Can you work these out from the model? Positions are in its coordinate system, mm. Coordinates: 2 decimals unless noted, no trailing zeros. Order: outer loops, then holes, each group sorted by start corner. A loop starts at its lowest first (then second) coordinate and runs counter-clockwise, first axis right, second up. Notation, with made-up numbers: (60.5, 1.25) -> (102.5, 1.25) arc R20 ccw to (102.5, 26.25) -> close; hole circle Ø9 at (64, 29.5). An arc over 180 degrees is marked (long way). Answer in a Markdown table with one row per item. Add a question column.
1. If I drill on line 1 along Y through (x, z) = (41.7, 1.6); line 2 along X through (y, z) = (5.5, 0.65); line 3 along Y through (x, z) = (42.5, 0.95), over which ranges is the centre line in solid material (lowest first)? Write a range as [from, to].
2. Imagine slicing it at C-C on x = 24. Write out the boundary of the cut face in (y, z), plus the area to 3 significant figures.
3. Imagine slicing it at D-D on z = 1.4. Write out the boundary of the cut face in (x, y), plus the area to 3 significant figures.
4. Imagine slicing it at B-B on x = 31.5. Write out the boundary of the cut face in (y, z).
5. Will these pins go through, and if not, where does the flat tip stop? pin 1 (1.5 mm diameter, centred on x = 5, y = 24.5, fed in from +Z); pin 2 (0.9 mm diameter, centred on x = 36.5, z = 2, fed in from -Y); pin 3 (1.5 mm diameter, centred on y = 30, z = 1, fed in from -X); pin 4 (1.5 mm diameter, centred on y = 21.5, z = 1.5, fed in from -X).
6. Imagine slicing it at A-A on x = 41.7. Write out the boundary of the cut face in (y, z).
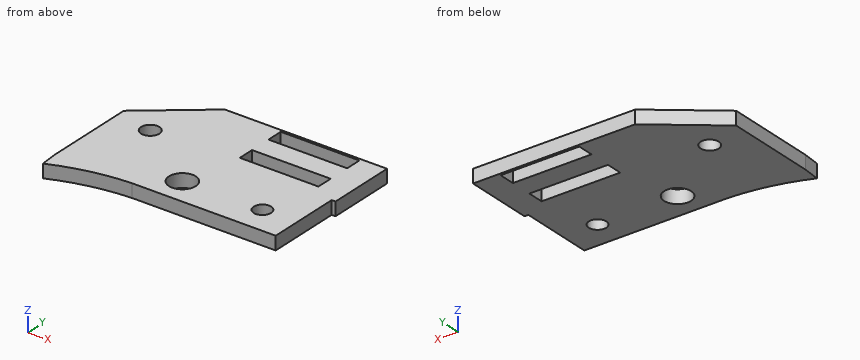
from build123d import *

# Parameters (mm, degrees)
SKETCH_1_R      = 3
SKETCH_1_R_2    = 1.95
SKETCH_1_R_3    = 2.05
SKETCH_1_W      = 17.535566723
SKETCH_1_H      = 3.6
EXTRUDE_1_DEPTH = 3


with BuildPart() as part:
    # 스케치1 → 보스-돌출1 (new body)
    with BuildSketch(Plane.XY):
        with BuildLine():
            Line((14.033980913, 31.631973376), (0, 20.408728084))
            Line((0, 20.408728084), (0, 0))
            Line((0, 0), (0.315433782, -3.780966668))
            ThreePointArc((0.315433782, -3.780966668), (8.660717355, -1.110252043), (17.352311853, 0))
            Line((17.352311853, 0), (49.356011681, 0))
            Line((49.356011681, 0), (49.356011681, 16.484705835))
            Line((49.356011681, 16.484705835), (50.213133896, 16.484705835))
            Line((50.213133896, 16.484705835), (50.213133896, 31.631973376))
            Line((50.213133896, 31.631973376), (14.033980913, 31.631973376))
        make_face()
        with Locations((24, 6)):
            Circle(SKETCH_1_R, mode=Mode.SUBTRACT)
        with Locations((41.7, 6.2)):
            Circle(SKETCH_1_R_2, mode=Mode.SUBTRACT)
        with Locations((8.103885944, 17.512168243)):
            Circle(SKETCH_1_R_3, mode=Mode.SUBTRACT)
        with Locations((35.691910847, 29.288073102)):
            Rectangle(SKETCH_1_W, SKETCH_1_H, mode=Mode.SUBTRACT)
        with Locations((35.691910847, 20.838073102)):
            Rectangle(SKETCH_1_W, SKETCH_1_H, mode=Mode.SUBTRACT)
    extrude(amount=EXTRUDE_1_DEPTH)


solid = part.part
Answers follow:
| question | item | result |
|---|---|---|
| 1 | line 1 | y = [0, 4.25], [8.15, 19.04], [22.64, 27.49], [31.09, 31.63] |
| 1 | line 2 | x = [0, 21.04], [26.96, 39.88], [43.52, 49.36] |
| 1 | line 3 | y = [0, 4.42], [7.98, 19.04], [22.64, 27.49], [31.09, 31.63] |
| 2 | outline | (0, 0) -> (3, 0) -> (3, 3) -> (0, 3) -> close; (9, 0) -> (31.63, 0) -> (31.63, 3) -> (9, 3) -> close |
| 2 | area | 76.9 mm² |
| 3 | outline | (0, 0) -> (0.32, -3.78) arc R48.03 cw to (17.35, 0) -> (49.36, 0) -> (49.36, 16.48) -> (50.21, 16.48) -> (50.21, 31.63) -> (14.03, 31.63) -> (0, 20.41) -> close; hole circle Ø4.1 at (8.1, 17.51); hole circle Ø6 at (24, 6); hole (26.92, 19.04) -> (44.46, 19.04) -> (44.46, 22.64) -> (26.92, 22.64) -> close; hole (26.92, 27.49) -> (44.46, 27.49) -> (44.46, 31.09) -> (26.92, 31.09) -> close; hole circle Ø3.9 at (41.7, 6.2) |
| 3 | area | 1,340 mm² |
| 4 | outline | (0, 0) -> (19.04, 0) -> (19.04, 3) -> (0, 3) -> close; (22.64, 0) -> (27.49, 0) -> (27.49, 3) -> (22.64, 3) -> close; (31.09, 0) -> (31.63, 0) -> (31.63, 3) -> (31.09, 3) -> close |
| 5 | pin 1 | stops at z = 3 |
| 5 | pin 2 | stops at y = 0 |
| 5 | pin 3 | stops at x = 11.06 |
| 5 | pin 4 | stops at x = 0.43 |
| 6 | outline | (0, 0) -> (4.25, 0) -> (4.25, 3) -> (0, 3) -> close; (8.15, 0) -> (19.04, 0) -> (19.04, 3) -> (8.15, 3) -> close; (22.64, 0) -> (27.49, 0) -> (27.49, 3) -> (22.64, 3) -> close; (31.09, 0) -> (31.63, 0) -> (31.63, 3) -> (31.09, 3) -> close |
